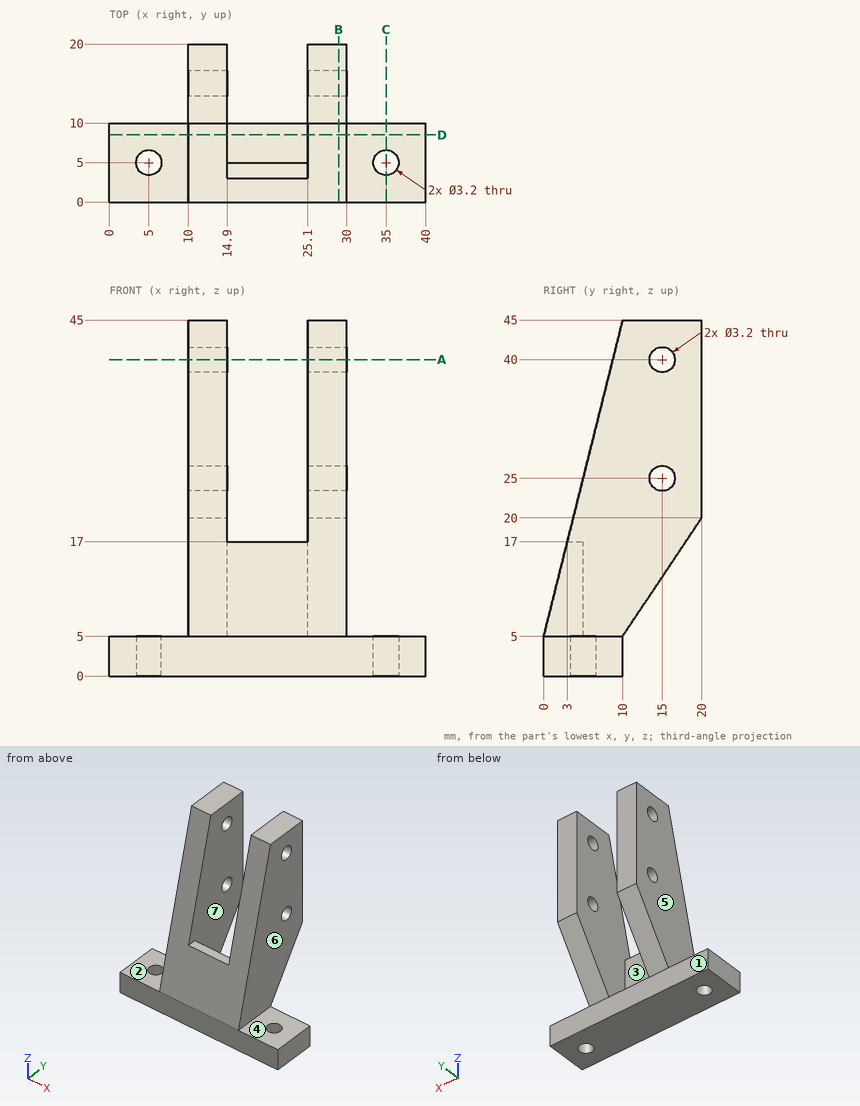
Here's the drawing with two shaded views (mm, measured from the low corner). I have some questions. A direction names the side the tool comes from. Round coordinates to 2 decimals unless told otherwise and drop trailing zeros. Loops run counter-clockwise (first coordinate to the right, second up) from the corner with the lowest first, then second, coordinate; pieces in that order, holes last. Notation, with made-up numbers: (20.5, -26) - (67.5, -26) arc R19 ccw to (67.5, -10) - close; hole circle Ø4 at (6.5, -31.75). An arc over 180 degrees is marked (long way). Write item = value, one per line.
1) If we mould it in two halves opening along X, with no side actions, what happens to the marked faces 4, 5, 6 and 7? For each: pulls with the +X half, pulls with the -X half, needs draft (parallel to the pull), parting line crosses it, or undercut.
Computed:
face_4 = needs draft
face_5 = pulls with the -X half
face_6 = pulls with the +X half
face_7 = undercut
2) Imagine slicing it at A-A (z = 40). Please give me the cut outline in (x, y).
Computed:
outline = (10, 8.75) - (14.9, 8.75) - (14.9, 13.4) - (10, 13.4) - close; (10, 16.6) - (14.9, 16.6) - (14.9, 20) - (10, 20) - close; (25.1, 8.75) - (30, 8.75) - (30, 13.4) - (25.1, 13.4) - close; (25.1, 16.6) - (30, 16.6) - (30, 20) - (25.1, 20) - close
3) Imagine slicing it at C-C (x = 35). Please give me the cut outline in (y, z).
Computed:
outline = (0, 0) - (3.4, 0) - (3.4, 5) - (0, 5) - close; (6.6, 0) - (10, 0) - (10, 5) - (6.6, 5) - close
4) I'm going to push flat-ended pins straight in: P1, Ø5, axis at y = 8.5, z = 34, coming from the -X side; P2, Ø6, axis at x = 22.5, z = 10.5, coming from the -Y side (3 decimals); P3, Ø5, axis at x = 35, y = 5, coming from the +Z side; P4, Ø2, axis at x = 19, y = 5.5, coming from the -Z side. Where does each tip first touch, or does it pass through?
Computed:
P1 = 10
P2 = 0.625
P3 = 5
P4 = 0
5) I need wall thicknesses on line 1 along X through (y, z) = (6, 21); line 2 along Y through (x, z) = (27, 25); line 3 along Y through (x, z) = (35, 3.05). Which ranges of each line are inside material? Lowest first, please. Write a range as from..to.
Computed:
line_1 = 10..14.9, 25.1..30
line_2 = 5..13.4, 16.6..20
line_3 = 0..3.4, 6.6..10
6) Imagine slicing it at B-B (x = 29). Please give me the cut outline in (y, z).
Computed:
outline = (0, 0) - (10, 0) - (10, 5) - (20, 20) - (20, 45) - (10, 45) - (0, 5) - close; hole circle Ø3.2 at (15, 25); hole circle Ø3.2 at (15, 40)
7) Imagine slicing it at D-D (y = 8.5). Please give me the cut outline in (x, z).
Computed:
outline = (0, 0) - (40, 0) - (40, 5) - (30, 5) - (30, 39) - (25.1, 39) - (25.1, 5) - (14.9, 5) - (14.9, 39) - (10, 39) - (10, 5) - (0, 5) - close
8) On a 3-axis mill with a long thin cutter (end or side, diameter ignored), from which of +Z, -Z, +X, -X, +Y, -Y can I reach the whole of each face in a straight line? I mean the marked faces 1, 2 and 3. Say none if no direction works.
Computed:
face_1 = -Z, +X, -X, +Y
face_2 = +Z, -X, +Y, -Y
face_3 = +Z, +Y
